Read the model definition and answer for the solid it produces. Units are mm, in the model's axes. Give positions to 0.01 mm unless a question says otherwise; leave off trailing zeros. Write each loop counter-clockwise with the first axis right and the second up, starting at its lowest first coordinate (ties: lowest second). Pieces come first, ordered by that corner, then holes.
```python
from build123d import *

# Parameters (mm, degrees)
SERVOSPLINEPROFILE_R = 3.362297175
SERVOKEY_DEPTH       = 5


with BuildPart() as part:
    # ServoSplineProfile → ServoKey (new body)
    with BuildSketch(Plane.XY):
        Circle(SERVOSPLINEPROFILE_R)
        Polygon((0.214716449, 2.628050171), (0.373952201, 2.361041273), (0.923370571, 2.841842406), (1.085251555, 2.129926103), (1.756355197, 2.41741554), (1.690318926, 1.690318926), (2.41741554, 1.756355197), (2.129926103, 1.085251555), (2.841842406, 0.923370571), (2.361041273, 0.373952201), (2.988089937, 0), (2.361041273, -0.373952201), (2.841842406, -0.923370571), (2.129926103, -1.085251555), (2.41741554, -1.756355197), (1.690318926, -1.690318926), (1.756355197, -2.41741554), (1.085251555, -2.129926103), (0.923370571, -2.841842406), (0.373952201, -2.361041273), (0, -2.988089937), (-0.373952201, -2.361041273), (-0.923370571, -2.841842406), (-1.085251555, -2.129926103), (-1.756355197, -2.41741554), (-1.690318926, -1.690318926), (-2.41741554, -1.756355197), (-2.129926103, -1.085251555), (-2.841842406, -0.923370571), (-2.361041273, -0.373952201), (-2.988089937, 0), (-2.361041273, 0.373952201), (-2.841842406, 0.923370571), (-2.129926103, 1.085251555), (-2.41741554, 1.756355197), (-1.690318926, 1.690318926), (-1.756355197, 2.41741554), (-1.085251555, 2.129926103), (-0.923370571, 2.841842406), (-0.373952201, 2.361041273), (-0.214716449, 2.628050171), (0, 2.988089937), align=None, mode=Mode.SUBTRACT)
    extrude(amount=SERVOKEY_DEPTH)


solid = part.part
```
Item 1: Find the intervals of material crossed by line 1 along Y through (x, z) = (-2.5, 2.6); line 2 along X through (y, z) = (2.25, 2.7); line 3 along Y through (x, z) = (0.75, 4.6), in increasing order.
Result set:
line 1: y = -2.25 to -1, -0.53 to -0.29, 0.29 to 0.53, 1 to 2.25
line 2: x = -2.5 to -1.74, -1.37 to -1.06, 1.06 to 1.37, 1.74 to 2.5
line 3: y = -3.28 to -2.69, 2.69 to 3.28
Item 2: Section A-A (x = -2) is taken. Write down the section's boundary in (y, z).
Result set:
outline: (-2.7, 0) - (-1.72, 0) - (-1.72, 5) - (-2.7, 5) - close; (1.72, 0) - (2.7, 0) - (2.7, 5) - (1.72, 5) - close
Item 3: Section C-C (x = -2.75) is taken. Write down the section's boundary in (y, z), and give its area (3 significant figures).
Result set:
outline: (-1.93, 0) - (-0.94, 0) - (-0.94, 5) - (-1.93, 5) - close; (-0.82, 0) - (-0.14, 0) - (-0.14, 5) - (-0.82, 5) - close; (0.14, 0) - (0.82, 0) - (0.82, 5) - (0.14, 5) - close; (0.94, 0) - (1.93, 0) - (1.93, 5) - (0.94, 5) - close
area: 16.7 mm2
Item 4: Each of these flat-tipped pins is pushed along its axis until it touches: pin 1 Ø2 at (x, y) = (0, -2.5) entering from +Z; pin 2 Ø3 at (x, z) = (-2, 3.5) entering from +Y. Where does it stop, or does it pass through?
Result set:
pin 1: stops at z = 5
pin 2: stops at y = 3.32
Item 5: Section B-B (y = 1.5) is taken. Write down the section's boundary in (x, z), and give its area (3 significant figures).
Result set:
outline: (-3.01, 0) - (-2.31, 0) - (-2.31, 5) - (-3.01, 5) - close; (2.31, 0) - (3.01, 0) - (3.01, 5) - (2.31, 5) - close
area: 7.02 mm2
